For this review, take the finished solid that the model builds, in its own axes (mm). Coordinates: 2 decimals unless noted, no trailing zeros. Loops run counter-clockwise (first coordinate to the right, second up) from the corner with the lowest first, then second, coordinate; pieces in that order, holes last.
1. Clearance check with flat-ended pins moving along their axes: P1, Ø1.1, axis at x = -0.5, z = -7, coming from the +Y side; P2, Ø0.6, axis at x = 7, z = 2, coming from the -Y side; P3, Ø1, axis at x = 2, z = 0, coming from the +Y side; P4, Ø3, axis at x = 2.5, y = -0.5, coming from the -Z side. State where each tip first meets the part, or that it passes through.
2. Take a section at A-A, the plane x = -1.75. State the section outline as (y, z) points.
3. Mouldability with a two-part tool opening along X and no side actions: class faces 1 (the face through (-6.84, -1.4, 0.984)), 2 (the face through (-6.74, -1.4, 2.93)), 3 (the face through (-1.32, -1.4, 6.77)), 4 (the face through (7.049, -1.4, 2.086)) as pulls with the +X half, pulls with the -X half, needs draft (parallel to the pull), parting line crosses it, or undercut.
4. To check wall thickness, follow probe 1 along Z at (x, y) = (0, -3.25); probe 2 along Z at (x, y) = (0, -1.5) (3 decimals); probe 3 along Z at (x, y) = (6.75, -2.1). State the ranges of each line that lie inside material, in increasing order.
```python
from build123d import *

# Parameters (mm, degrees)
F0_R     = 6.435
F0_R_2   = 4.08
F1_DEPTH = 5.7
F3_DEPTH = 2.85
F5_DEPTH = 2.84


with BuildPart() as f1:
    # F0 (on Front) → F1 (new body)
    with BuildSketch(Plane.XZ):
        Circle(F0_R)
        Circle(F0_R_2, mode=Mode.SUBTRACT)
    extrude(amount=F1_DEPTH)

    # F2 (on face) → F3 (join)
    with BuildSketch(Plane.XZ.offset(5.7)):
        Polygon((-2.59842, 6.898823), (-2.334261, 5.996703), (-1.268992, 6.308636), (-1.53315, 7.210756), align=None)
        Polygon((-0.109072, 7.371136), (-0.165965, 6.432859), (0.942, 6.365678), (0.998893, 7.303955), align=None)
        Polygon((-4.821629, 5.576508), (-4.262099, 4.821176), (-3.370165, 5.481899), (-3.929696, 6.23723), align=None)
        Polygon((-5.642754, 3.093308), (-5.027217, 4.017003), (-5.809446, 4.538269), (-6.424983, 3.614573), align=None)
        Polygon((-7.278092, 1.172569), (-6.363949, 0.953611), (-6.105393, 2.033078), (-7.019536, 2.252036), align=None)
        Polygon((-6.31094, -1.257481), (-6.433151, -0.15423), (-7.367437, -0.257724), (-7.245225, -1.360976), align=None)
        Polygon((-6.329055, -3.780028), (-5.488037, -3.360159), (-5.983839, -2.367043), (-6.824857, -2.786911), align=None)
        Polygon((-4.026167, -5.019881), (-4.828943, -4.253297), (-5.478122, -4.933125), (-4.675346, -5.699709), align=None)
        Polygon((-2.418582, -6.963907), (-2.044212, -6.101674), (-3.062381, -5.659598), (-3.436752, -6.521831), align=None)
        Polygon((0.142494, -6.433422), (-0.965218, -6.362199), (-1.025533, -7.300262), (0.082179, -7.371485), align=None)
        Polygon((2.623572, -6.889297), (2.356123, -5.988147), (1.291999, -6.303964), (1.559448, -7.205114), align=None)
        Polygon((4.244481, -4.836694), (3.350143, -5.494158), (3.906914, -6.251525), (4.801252, -5.594061), align=None)
        Polygon((6.438127, -3.591109), (5.654002, -3.0727), (5.041839, -3.998636), (5.825964, -4.517044), align=None)
        Polygon((6.360428, -0.976823), (6.097935, -2.055339), (7.011273, -2.27763), (7.273766, -1.199114), align=None)
        Polygon((7.240212, 1.3874), (6.30631, 1.280498), (6.432546, 0.177699), (7.366447, 0.284601), align=None)
        Polygon((5.50026, 3.340115), (5.992435, 2.345196), (6.834979, 2.761993), (6.342804, 3.756912), align=None)
        Polygon((4.654521, 5.716728), (4.007826, 5.034536), (4.813393, 4.270886), (5.460088, 4.953078), align=None)
        Polygon((2.066459, 6.094175), (3.083009, 5.648387), (3.460523, 6.509249), (2.443973, 6.955037), align=None)
    extrude(amount=-F3_DEPTH)

    # F4 (on face) → F5 (join)
    with BuildSketch(Plane(origin=(0, 0, 0), x_dir=(-1, 0, 0), z_dir=(0, 1, 0))):
        Polygon((-2.286011, 7.008294), (-2.065255, 6.094583), (-0.945089, 6.365221), (-1.165845, 7.278931), align=None)
        Polygon((0.270964, 7.366962), (0.165791, 6.432864), (1.268821, 6.30867), (1.373994, 7.242768), align=None)
        Polygon((-6.256031, 3.899245), (-5.4996, 3.341202), (-4.815465, 4.26855), (-5.571896, 4.826594), align=None)
        Polygon((-4.527821, 5.817592), (-4.007962, 5.034428), (-3.083161, 5.648304), (-3.603021, 6.431469), align=None)
        Polygon((-7.298784, -1.034304), (-6.360621, -0.975566), (-6.432631, 0.174578), (-7.370794, 0.11584), align=None)
        Polygon((-7.207989, 1.546107), (-6.306345, 1.280327), (-5.992499, 2.345034), (-6.894142, 2.610814), align=None)
        Polygon((-4.926355, -5.483891), (-4.245437, -4.835855), (-5.039898, -4.001081), (-5.720816, -4.649117), align=None)
        Polygon((-6.515458, -3.448819), (-5.653919, -3.072853), (-6.097879, -2.055504), (-6.959418, -2.43147), align=None)
        Polygon((-0.24883, -7.367504), (-0.143766, -6.433394), (-1.288941, -6.30459), (-1.394005, -7.2387), align=None)
        Polygon((-2.774272, -6.830004), (-2.355962, -5.988211), (-3.349994, -5.494248), (-3.768305, -6.336042), align=None)
        Polygon((4.545126, -5.80378), (4.025175, -5.020676), (3.065127, -5.658111), (3.585077, -6.441215), align=None)
        Polygon((2.265026, -7.015355), (2.044377, -6.101619), (0.96539, -6.362173), (1.18604, -7.275909), align=None)
        Polygon((7.212366, -1.524403), (6.310692, -1.258729), (5.984987, -2.364139), (6.886662, -2.629814), align=None)
        Polygon((6.244494, -3.918143), (5.488128, -3.360011), (4.829058, -4.253166), (5.585424, -4.811298), align=None)
        Polygon((6.50486, 3.468259), (5.643365, 3.092192), (6.104406, 2.03604), (6.965901, 2.412106), align=None)
        Polygon((7.302093, 1.012412), (6.363924, 0.953783), (6.433156, -0.154056), (7.371325, -0.095427), align=None)
        Polygon((2.753658, 6.838084), (2.335446, 5.996242), (3.367505, 5.483533), (3.785717, 6.325375), align=None)
        Polygon((4.942962, 5.469248), (4.261968, 4.821291), (5.027108, 4.017139), (5.708102, 4.665095), align=None)
    extrude(amount=-F5_DEPTH)


solid = f1.part
```
Results list:
1. P1: stops at y = -2.85
1. P2: stops at y = -2.84
1. P3: passes through
1. P4: stops at z = -7.28
2. outline: (-5.7, -6.19) - (-2.84, -6.19) - (-2.84, -7.14) - (0, -7.14) - (0, -3.69) - (-5.7, -3.69) - close; (-5.7, 3.69) - (0, 3.69) - (0, 6.19) - (-2.85, 6.19) - (-2.85, 7.15) - (-5.7, 7.15) - close
3. face 1: undercut
3. face 2: pulls with the -X half
3. face 3: undercut
3. face 4: pulls with the +X half
4. probe 1: z = -7.37 to -4.08, 4.08 to 7.36
4. probe 2: z = -6.435 to -4.08, 4.08 to 6.435
4. probe 3: z = -2.91 to -2.34, -1 to 0.15, 1.41 to 2.57
